```python
from build123d import *

# Parameters (mm, degrees)
SKETCH1_R               = 15.82
BOSS_EXTRUDE1_DEPTH     = 8.5
SKETCH2_R               = 12.615
BOSS_EXTRUDE2_DEPTH     = 11.4
SKETCH3_R               = 8.075
CUT_EXTRUDE1_DEPTH      = 30.942524944
CUT_EXTRUDE2_DEPTH      = 30.942524944
CUT_EXTRUDE2_DEPTH_BACK = 30.942524944
SKETCH4_R               = 2.1


with BuildPart() as part:
    # Sketch1 → Boss-Extrude1 (new body)
    with BuildSketch(Plane(origin=(0, 0, 0), x_dir=(0, 1, 0), z_dir=(0, 0, 1))):
        with Locations(Location((0, 0, 0), (0, 0, 270))):
            Circle(SKETCH1_R)
    extrude(amount=BOSS_EXTRUDE1_DEPTH)

    # Sketch2 → Boss-Extrude2 (add)
    with BuildSketch(Plane.XY.offset(8.5)):
        Circle(SKETCH2_R)
    extrude(amount=BOSS_EXTRUDE2_DEPTH)

    # Sketch3 → Cut-Extrude1 (cut, through all)
    with BuildSketch(Plane.XY.offset(19.9)):
        Circle(SKETCH3_R)
    extrude(amount=-CUT_EXTRUDE1_DEPTH, mode=Mode.SUBTRACT)

    # Sketch4 → Cut-Extrude2 (cut, two sides: drawn at the far end of the back side and taken through both)
    with BuildSketch(Plane(origin=(0, 0, 0), x_dir=(-1, 0, 0), z_dir=(0, 1, 0)).offset(-CUT_EXTRUDE2_DEPTH_BACK)):
        with Locations(Location((0, 14.2, 0), (0, 0, 90))):
            Circle(SKETCH4_R)
    extrude(amount=CUT_EXTRUDE2_DEPTH + CUT_EXTRUDE2_DEPTH_BACK, mode=Mode.SUBTRACT)


solid = part.part
```
The model under review builds one solid part; all positions refer to its coordinate system, in mm. A direction names the side the tool comes from. Round coordinates to 2 decimals unless told otherwise and drop trailing zeros. Order: outer loops, then holes, each group sorted by start corner. A loop starts at its lowest first (then second) coordinate and runs counter-clockwise, first axis right, second up. Notation, with made-up numbers: (-2.5, 25.5) -> (44.5, 25.5) arc R21 ccw to (44.5, 62.5) -> close; hole circle Ø2 at (59.25, -22). An arc over 180 degrees is marked (long way). One line per item, written item: value. Start each with the question number.
Q1. Machinability: for faces 1 (the face through (-0.18, -8.23, 19.9)), 2 (the face through (-2.735, -12.315, 14.12)), which of the approach directions +Z, -Z, +X, -X, +Y, -Y give a long, thin tool a straight path to every point of the face, cutting with its end or side? Answer none if there is none.
Q2. Mouldability with a two-part tool opening along X and no side actions: class faces 3 (the face through (0.09, 10.17, 12.1)), 4 (the face through (-11, -7, 8.5)), 5 (the face through (15.09, 4.75, 4.19)) as released by +X, released by -X, zero draft, split by the parting line, or undercut.
Q3. Take a section at B-B (x = 0). Write out the cut boundary in (y, z) (3 decimals).
Q4. Clearance check with flat-ended pins moving along their axes: pin 1 Ø6 at (y, z) = (3.5, 17.5) entering from -X; pin 2 Ø1 at (y, z) = (-7.5, 18) entering from +X; pin 3 Ø1.5 at (x, z) = (-0.5, 3) entering from -Y; pin 4 Ø8 at (x, z) = (-3.5, 17) entering from -Y (3 decimals). State where each tip first meets the part, or that it passes through.
Q5. Take a section at D-D (y = 9.5). Write out the cut boundary in (x, z), and give its area (3 significant figures).
Q6. Take a section at A-A (y = 0). Write out the cut boundary in (x, z) (3 decimals), and give its area (3 significant figures).
Q7. Take a section at C-C (z = 12.5). Write out the cut boundary in (x, y) (3 decimals), and give its area (3 significant figures).
Q8. Wall thickness on line 1 (Z direction, x = 0, y = -10.75); line 2 (Y direction, x = 5.5, z = 18.5); line 3 (Y direction, x = 1, z = 5.5): over which ranges is each line inside the solid? List them lowest first.
Reported:
1. face 1: +Z, +X, -X, +Y, -Y
1. face 2: +Z
2. face 3: undercut
2. face 4: zero draft
2. face 5: split by the parting line
3. outline: (-15.82, 0) -> (-8.075, 0) -> (-8.075, 12.1) -> (-12.615, 12.1) -> (-12.615, 8.5) -> (-15.82, 8.5) -> close; (-12.615, 16.3) -> (-8.075, 16.3) -> (-8.075, 19.9) -> (-12.615, 19.9) -> close; (8.075, 0) -> (15.82, 0) -> (15.82, 8.5) -> (12.615, 8.5) -> (12.615, 12.1) -> (8.075, 12.1) -> close; (8.075, 16.3) -> (12.615, 16.3) -> (12.615, 19.9) -> (8.075, 19.9) -> close
4. pin 1: stops at x = -12.61
4. pin 2: stops at x = 10.49
4. pin 3: stops at y = -15.82
4. pin 4: stops at y = -12.615
5. outline: (-12.65, 0) -> (12.65, 0) -> (12.65, 8.5) -> (8.3, 8.5) -> (8.3, 19.9) -> (-8.3, 19.9) -> (-8.3, 8.5) -> (-12.65, 8.5) -> close; hole circle Ø4.2 at (0, 14.2)
5. area: 390 mm2
6. outline: (-15.82, 0) -> (-8.075, 0) -> (-8.075, 19.9) -> (-12.615, 19.9) -> (-12.615, 8.5) -> (-15.82, 8.5) -> close; (8.075, 0) -> (15.82, 0) -> (15.82, 8.5) -> (12.615, 8.5) -> (12.615, 19.9) -> (8.075, 19.9) -> close
6. area: 235 mm2
7. outline: (-1.233, -12.555) -> (-1.233, -7.98) arc R8.075 cw to (-1.233, 7.98) -> (-1.233, 12.555) arc R12.615 ccw to start; (1.233, -12.555) arc R12.615 ccw to (1.233, 12.555) -> (1.233, 7.98) arc R8.075 cw to (1.233, -7.98) -> close
7. area: 273 mm2
8. line 1: z = 0 to 12.1, 16.3 to 19.9
8. line 2: y = -11.35 to -5.91, 5.91 to 11.35
8. line 3: y = -15.79 to -8.01, 8.01 to 15.79
